Read the model definition and answer for the solid it produces. Units are mm, in the model's axes. A direction names the side the tool comes from. Coordinates: 2 decimals unless noted, no trailing zeros. Order: outer loops, then holes, each group sorted by start corner. A loop starts at its lowest first (then second) coordinate and runs counter-clockwise, first axis right, second up. Notation, with made-up numbers: (-21.5, 30) - (-8.5, 30) arc R11 cw to (-8.5, 43) - close; hole circle Ø5 at (-20, -36.75). An arc over 180 degrees is marked (long way). Answer as a JSON object with one key per item and string values. Group by question number.
from build123d import *

# Parameters (mm, degrees)
F0_W     = 20.32
F0_H     = 42.8552175019
F0_W_2   = 18.5010901187
F1_DEPTH = 50.8


with BuildPart() as f1:
    # F0 (on Front) → F1 (new body)
    with BuildSketch(Plane.XZ):
        with BuildLine():
            Line((19.7615846992, 50.0709023562), (10.9937762186, 53.6630048046))
            ThreePointArc((10.9937762186, 53.6630048046), (9.505878667, 50.0709023562), (5.9137762186, 48.5830048046))
            Line((5.9137762186, 48.5830048046), (-1.7062237814, 48.5830048046))
            Line((-1.7062237814, 48.5830048046), (-9.3262237814, 48.5830048046))
            ThreePointArc((-9.3262237814, 48.5830048046), (-12.9183262298, 50.0709023562), (-14.4062237814, 53.6630048046))
            Line((-14.4062237814, 53.6630048046), (-21.1631003767, 50.0709023562))
            Line((-21.1631003767, 50.0709023562), (-24.4459839703, 47.2041854043))
            Line((-24.4459839703, 47.2041854043), (-24.4459839703, 25.8544358869))
            Line((-24.4459839703, 25.8544358869), (-24.4459839703, -16.4229627699))
            Line((-24.4459839703, -16.4229627699), (-20.7482980642, -16.4229627699))
            Line((-20.7482980642, -16.4229627699), (-0.4282980642, -16.4229627699))
            Line((-0.4282980642, -16.4229627699), (3.6740194462, -16.4229627699))
            Line((3.6740194462, -16.4229627699), (22.1751095649, -16.4229627699))
            Line((22.1751095649, -16.4229627699), (22.2648918826, -16.4229627699))
            Line((22.2648918826, -16.4229627699), (22.2648918826, 25.8544358869))
            Line((22.2648918826, 25.8544358869), (22.2648918826, 47.2041854043))
            Line((22.2648918826, 47.2041854043), (19.7615846992, 50.0709023562))
        make_face()
        with BuildLine():
            Line((23.3347140718, 47.2041854043), (22.2648918826, 47.2041854043))
            Line((22.2648918826, 47.2041854043), (22.2648918826, 25.8544358869))
            Line((22.2648918826, 25.8544358869), (23.3347140718, 25.8544358869))
            ThreePointArc((23.3347140718, 25.8544358869), (24.7715550512, 26.4495949076), (25.3667140718, 27.8864358869))
            Line((25.3667140718, 27.8864358869), (25.3667140718, 45.1721854043))
            ThreePointArc((25.3667140718, 45.1721854043), (24.7715550512, 46.6090263836), (23.3347140718, 47.2041854043))
        make_face()
        Polygon((56.5698947954, 6.5076726805), (25.3667140718, 45.1721854043), (25.3667140718, 27.8864358869), (48.6546903849, 0), (52.1676763892, 2.9549777973), align=None)
        with BuildLine():
            Line((62.7134148699, -0.7986944953), (56.5698947954, 6.5076726805))
            Line((56.5698947954, 6.5076726805), (52.1676763892, 2.9549777973))
            Line((52.1676763892, 2.9549777973), (48.6546903849, 0))
            Line((48.6546903849, 0), (54.4804789865, -7.2188562926))
            ThreePointArc((54.4804789865, -7.2188562926), (61.7538678556, -8.0570733036), (62.7134148699, -0.7986944953))
        make_face()
        with BuildLine():
            Line((-24.4459839703, 25.8544358869), (-24.4459839703, 47.2041854043))
            Line((-24.4459839703, 47.2041854043), (-25.5158065703, 47.2041854043))
            ThreePointArc((-25.5158065703, 47.2041854043), (-26.9526475496, 46.6090263836), (-27.5478065703, 45.1721854043))
            Line((-27.5478065703, 45.1721854043), (-27.5478065703, 27.8864358869))
            ThreePointArc((-27.5478065703, 27.8864358869), (-26.9526475496, 26.4495949076), (-25.5158065703, 25.8544358869))
            Line((-25.5158065703, 25.8544358869), (-24.4459839703, 25.8544358869))
        make_face()
        Polygon((-27.5478065703, 27.8864358869), (-27.5478065703, 45.1721854043), (-59.8365601521, 6.5076726805), (-50.8357828875, 0), align=None)
        with BuildLine():
            Line((-50.8357828875, 0), (-59.8365601521, 6.5076726805))
            Line((-59.8365601521, 6.5076726805), (-63.5941543789, 1.4677946764))
            ThreePointArc((-63.5941543789, 1.4677946764), (-64.5350303405, -2.3878407212), (-62.4158617427, -5.7434772254))
            Line((-62.4158617427, -5.7434772254), (-61.8365846936, -6.1450817318))
            ThreePointArc((-61.8365846936, -6.1450817318), (-58.0368035716, -6.9689157861), (-54.7674139269, -4.8646034341))
            Line((-54.7674139269, -4.8646034341), (-56.3995838165, -7.2188562926))
            Line((-56.3995838165, -7.2188562926), (-50.8357828875, 0))
        make_face()
        with Locations((-10.5882980642, -37.8505715208)):
            Rectangle(F0_W, F0_H)
        with Locations((12.9245645056, -37.8505715208)):
            Rectangle(F0_W_2, F0_H)
        with BuildLine():
            Line((23.3365580372, -59.2781802717), (22.1751095649, -59.2781802717))
            Line((22.1751095649, -59.2781802717), (3.6740194462, -59.2781802717))
            Line((3.6740194462, -59.2781802717), (1.3876754092, -59.2781802717))
            Line((1.3876754092, -59.2781802717), (1.3876754092, -73.2621923089))
            Line((1.3876754092, -73.2621923089), (28.4165580372, -73.2621923089))
            Line((28.4165580372, -73.2621923089), (28.4165580372, -64.3581802717))
            ThreePointArc((28.4165580372, -64.3581802717), (26.9286604856, -60.7660778233), (23.3365580372, -59.2781802717))
        make_face()
        with BuildLine():
            Line((0, -59.2781802717), (-0.4282980642, -59.2781802717))
            Line((-0.4282980642, -59.2781802717), (-20.7482980642, -59.2781802717))
            Line((-20.7482980642, -59.2781802717), (-26.2982390387, -59.2781802717))
            ThreePointArc((-26.2982390387, -59.2781802717), (-26.6574492835, -59.4269700269), (-26.8062390387, -59.7861802717))
            Line((-26.8062390387, -59.7861802717), (-26.8062390387, -73.2621923089))
            Line((-26.8062390387, -73.2621923089), (0, -73.2621923089))
            Line((0, -73.2621923089), (0, -59.7561709583))
            Line((0, -59.7561709583), (0, -59.2781802717))
        make_face()
        with BuildLine():
            ThreePointArc((5.9137762186, 48.5830048046), (9.505878667, 50.0709023562), (10.9937762186, 53.6630048046))
            Line((10.9937762186, 53.6630048046), (10.9937762186, 55.117353797))
            Line((10.9937762186, 55.117353797), (10.9937762186, 58.5980406803))
            Line((10.9937762186, 58.5980406803), (10.9937762186, 62.3222826543))
            Line((10.9937762186, 62.3222826543), (10.9937762186, 65.9971610492))
            ThreePointArc((10.9937762186, 65.9971610492), (7.2740323397, 74.9774171703), (-1.7062237814, 78.6971610492))
            ThreePointArc((-1.7062237814, 78.6971610492), (-10.6864799025, 74.9774171703), (-14.4062237814, 65.9971610492))
            Line((-14.4062237814, 65.9971610492), (-14.4062237814, 62.3222826543))
            Line((-14.4062237814, 62.3222826543), (-14.4062237814, 58.5980406803))
            Line((-14.4062237814, 58.5980406803), (-14.4062237814, 55.117353797))
            Line((-14.4062237814, 55.117353797), (-14.4062237814, 53.6630048046))
            ThreePointArc((-14.4062237814, 53.6630048046), (-12.9183262298, 50.0709023562), (-9.3262237814, 48.5830048046))
            Line((-9.3262237814, 48.5830048046), (-1.7062237814, 48.5830048046))
            Line((-1.7062237814, 48.5830048046), (5.9137762186, 48.5830048046))
        make_face()
    extrude(amount=F1_DEPTH)


solid = f1.part
1. Straight lines are drawn through the part: L1, parallel to X at y = -23, z = -30; L2, parallel to X at y = -5, z = -3; L3, parallel to X at y = -20, z = 13. For each, find the intervals that lie inside material, in ascending order.
2. For faces 1 (the cylindrical face through (26.97, -25.04, -60.81)), 2 (the flat face through (-0.428, -25, -38)), 3 (the flat face through (-53.657, -25.044, -3.66)), 4 (the flat face through (-23, -25, -16.423)), determine the directions among +Z, -Z, +X, -X, +Y, -Y from which every point of the face is accessible in a straight line to the end or side of a thin tool.
3. A cutting plane is placed at A-A on z = -41. Write down the section's boundary in (x, y).
4. A cutting plane is placed at B-B on x = -11. Write down the section's boundary in (y, z), and give its area (3 significant figures).
5. For a pull along Z with two mould halves and no side action, classify faces 5 (the cylindrical face through (61.7, -25, -8.1)), 6 (the flat face through (59.685, -25.044, 2.803)), 7 (the flat face through (22.265, -25, 4)) as pulls with the +Z half, pulls with the -Z half, needs draft (parallel to the pull), parting line crosses it, or undercut.
6. A cutting plane is placed at C-C on z = 39.5. Write down the section's boundary in (x, y), and give its area (3 significant figures).
7. Given pin 1 (12 mm diameter, centred on y = -30.5, z = 31, fed in from +X); pin 2 (6 mm diameter, centred on x = 25, z = -36, fed in from +Y); pin 3 (13 mm diameter, centred on y = -25.5, z = -32.5, fed in from -X); pin 4 (8 mm diameter, centred on y = -39.5, z = 60.5, fed in from -X), each flat-ended and moving along its own axis, determine where each tip first touches the part or whether it passes through.
Derived:
{
 "1": {"L1": "x = -20.75 to -0.43, 3.67 to 22.18", "L2": "x = -64.4 to -53.15, -24.45 to 22.26, 51.08 to 63.68", "L3": "x = -54.41 to -39.98, -24.45 to 22.26, 37.8 to 51.33"},
 "2": {"face 1": "+X, +Y, -Y", "face 2": "+Y, -Y", "face 3": "-Z, +Y, -Y", "face 4": "-X, +Y, -Y"},
 "3": {"outline": "(-20.75, -50.8) - (-0.43, -50.8) - (-0.43, 0) - (-20.75, 0) - close; (3.67, -50.8) - (22.18, -50.8) - (22.18, 0) - (3.67, 0) - close"},
 "4": {"outline": "(-50.8, -73.26) - (0, -73.26) - (0, 74.65) - (-50.8, 74.65) - close", "area": "7,510 mm2"},
 "5": {"face 5": "parting line crosses it", "face 6": "pulls with the +Z half", "face 7": "undercut"},
 "6": {"outline": "(-32.28, -50.8) - (29.94, -50.8) - (29.94, 0) - (-32.28, 0) - close", "area": "3,160 mm2"},
 "7": {"pin 1": "stops at x = 41.65", "pin 2": "stops at y = 0", "pin 3": "stops at x = -20.75", "pin 4": "stops at x = -14.41"}
}
